Here's how the part is built. I have some questions about the finished solid (model axes, mm). A direction names the side the tool comes from. Round coordinates to 2 decimals unless told otherwise and drop trailing zeros. Order: outer loops, then holes, each group sorted by start corner. A loop starts at its lowest first (then second) coordinate and runs counter-clockwise, first axis right, second up. Notation, with made-up numbers: M 8,-40 L 32,-40 A19 ccw 32,-16 Z; hole C 46.25,74.25 d1. An arc over 180 degrees is marked long. Write item = value, one per line. Start each with the question number.
Item 1: Please list where these lines run through material, in increasing order: L1, parallel to Z at x = 0, y = 9.9; L2, parallel to X at y = 9.85, z = 0; L3, parallel to X at y = 9.1, z = 0.
Item 2: We'd pull the mould along Z, two halves only. Please class faces 1 (the face through (-23.671, 6.306, -1.042)), 2 (the face through (7, 12, 20)), 3 (the face through (-18.936, 11.139, 14.519)): pulls with the +Z half, pulls with the -Z half, needs draft (parallel to the pull), parting line crosses it, or undercut.
Item 3: I want a section at A-A, the plane x = 0. List the corners of the cut face in (y, z) for me, plus the area to 3 significant figures.
Item 4: I want a section at C-C, the plane y = 2.5. List the corners of the cut face in (x, z) for me.
Item 5: I want a section at D-D, the plane y = 10. List the corners of the cut face in (x, z) for me, plus the area to 3 significant figures.
Item 6: For faces 4 (the face through (-4.336, 9.479, 19.524)), 5 (the face through (-20, 7, 7)), which set-ups out of +Z, -Z, +X, -X, +Y, -Y let a thin tool reach every point of the face, with its end or its side?
Item 7: I'm going to push flat-ended pins straight in: P1, Ø1.5, axis at x = -25, z = -11, coming from the +Y side; P2, Ø3, axis at x = 24, z = -16.5, coming from the -Y side; P3, Ø2, axis at y = 10.5, z = -22, coming from the -X side; P4, Ø3, axis at y = 6.5, z = -7.5, coming from the -X side. Where does each tip first touch, or does it pass through?
Item 8: I want a section at B-B, the plane z = 0. List the corners of the cut face in (x, y) for me, plus the area to 3 significant figures.
```python
from build123d import *

# Parameters (mm, degrees)
FILLET_R = 1


with BuildPart() as part:
    # Sketch → Revolution (revolve)
    with BuildSketch(Plane.XY):
        Polygon((20, 7), (23, 7), (30, 0), (35, 0), (23, 12), (20, 12), align=None)
    revolve(axis=Axis((0, 0, 0), (0, 1, 0)))

    # Fillet
    fillet_edges = [part.edges().sort_by_distance(p)[0] for p in [
        (-30, 0, 0),
        (-23, 7, 0),
        (-20, 7, 0),
        (-23, 12, 0),
        (-20, 12, 0),
    ]]
    fillet(fillet_edges, radius=FILLET_R)


solid = part.part
```
Filled in:
q1.L1 = -25.1 to -20, 20 to 25.1
q1.L2 = -25.15 to -20, 20 to 25.15
q1.L3 = -25.9 to -20, 20 to 25.9
q2.face_1 = undercut
q2.face_2 = needs draft
q2.face_3 = parting line crosses it
q3.outline = M 0,-35 L 11.71,-23.29 A1 ccw 12,-22.59 L 12,-21 A1 ccw 11,-20 L 8,-20 A1 ccw 7,-21 L 7,-22.59 A1 cw 6.71,-23.29 L 0.29,-29.71 A1 ccw 0,-30.41 Z; M 0,30.41 A1 ccw 0.29,29.71 L 6.71,23.29 A1 cw 7,22.59 L 7,21 A1 ccw 8,20 L 11,20 A1 ccw 12,21 L 12,22.59 A1 ccw 11.71,23.29 L 0,35 Z
q3.area = 124 mm^2
q4.outline = C 0,0 d65; hole C 0,0 d55
q5.outline = C 0,0 d50; hole C 0,0 d40
q5.area = 707 mm^2
q6.face_4 = +Y, -Y
q6.face_5 = -Y
q7.P1 = 8.44
q7.P2 = 0
q7.P3 = -13.5
q7.P4 = -29.09
q8.outline = M -35,0 L -30.41,0 A1 ccw -29.71,0.29 L -23.29,6.71 A1 cw -22.59,7 L -21,7 A1 ccw -20,8 L -20,11 A1 ccw -21,12 L -22.59,12 A1 ccw -23.29,11.71 Z; M 20,8 A1 ccw 21,7 L 22.59,7 A1 cw 23.29,6.71 L 29.71,0.29 A1 ccw 30.41,0 L 35,0 L 23.29,11.71 A1 ccw 22.59,12 L 21,12 A1 ccw 20,11 Z
q8.area = 124 mm^2
